Geometry check sheet. Reference: drawing and pictorial views, mm from the part's lowest x, y, z. A direction names the side the tool comes from. Give positions to 0.01 mm unless a question says otherwise; leave off trailing zeros. Order: outer loops, then holes, each group sorted by start corner. A loop starts at its lowest first (then second) coordinate and runs counter-clockwise, first axis right, second up. Notation, with made-up numbers: (49.5, 2) - (75.5, 2) arc R24 ccw to (75.5, 25) - close; hole circle Ø9 at (7, 50). An arc over 180 degrees is marked (long way). Answer as a JSON object with one key per item and string values.
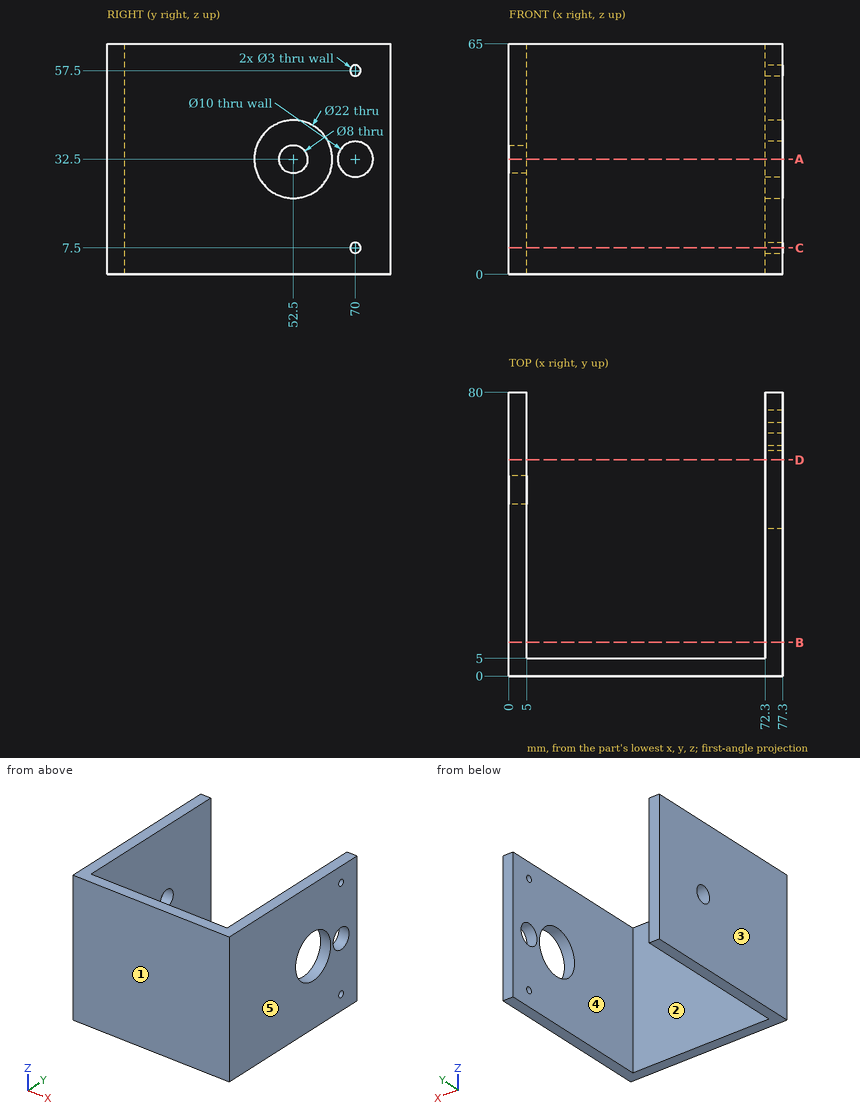
(1) Section check A-A (z = 32.5). Record the cut outline in (x, y), then the cut area to 4 significant figures.
Computed values:
{"outline": "(0, 0) - (77.3, 0) - (77.3, 41.5) - (72.3, 41.5) - (72.3, 5) - (5, 5) - (5, 48.5) - (0, 48.5) - close; (0, 56.5) - (5, 56.5) - (5, 80) - (0, 80) - close; (72.3, 63.5) - (77.3, 63.5) - (77.3, 65) - (72.3, 65) - close; (72.3, 75) - (77.3, 75) - (77.3, 80) - (72.3, 80) - close", "area": "936.5 mm²"}
(2) Section check D-D (y = 61). Record the cut outline in (x, z).
Computed values:
{"outline": "(0, 0) - (5, 0) - (5, 65) - (0, 65) - close; (72.3, 0) - (77.3, 0) - (77.3, 25.52) - (72.3, 25.52) - close; (72.3, 39.48) - (77.3, 39.48) - (77.3, 65) - (72.3, 65) - close"}
(3) Gauge pin test, flat ends, axial feed: pin 1 Ø6 at (y, z) = (70, 32.5) entering from +X; pin 2 Ø2 at (x, z) = (58.5, 30.5) entering from +Y. Record the tip position at first contact, or that the pin passes through.
Computed values:
{"pin 1": "stops at x = 5", "pin 2": "stops at y = 5"}
(4) Section check B-B (y = 9.5). Record the cut outline in (x, z), then the cut area to 3 significant figures.
Computed values:
{"outline": "(0, 0) - (5, 0) - (5, 65) - (0, 65) - close; (72.3, 0) - (77.3, 0) - (77.3, 65) - (72.3, 65) - close", "area": "650 mm²"}
(5) Access from +Z, -Z, +X, -X, +Y, -Y to the whole of each face (thin tool, end or side, straight path). Record for the marked faces 4 and 5.
Computed values:
{"face 4": "+Z, -Z, +Y", "face 5": "+Z, -Z, +X, +Y, -Y"}
(6) Section check C-C (z = 7.5). Record the cut outline in (x, y).
Computed values:
{"outline": "(0, 0) - (77.3, 0) - (77.3, 68.5) - (72.3, 68.5) - (72.3, 5) - (5, 5) - (5, 80) - (0, 80) - close; (72.3, 71.5) - (77.3, 71.5) - (77.3, 80) - (72.3, 80) - close"}
(7) Release check for a two-part mould opening along X. For the marked faces 1, 2 and 3 record: pulls with the +X half, pulls with the -X half, needs draft (parallel to the pull), parting line crosses it, or undercut.
Computed values:
{"face 1": "needs draft", "face 2": "undercut", "face 3": "pulls with the -X half"}
(8) Material ranges on line 1 along Y through (x, z) = (74.3, 32.5); line 2 along X through (y, z) = (66, 17.5); line 3 along Y through (x, z) = (2.45, 32.5), recorded low to high. Write a range as [from, to].
Computed values:
{"line 1": "y = [0, 41.5], [63.5, 65], [75, 80]", "line 2": "x = [0, 5], [72.3, 77.3]", "line 3": "y = [0, 48.5], [56.5, 80]"}
